Input: part model. Units: mm. Frame: model coordinates. Face numbers are marked on the shaded views. A direction names the side the tool comes from. Give positions to 0.01 mm unless a question says otherwise; leave off trailing zeros. Write each loop counter-clockwise with the first axis right and the second up, starting at its lowest first coordinate (ties: lowest second). Pieces come first, ordered by that corner, then holes.
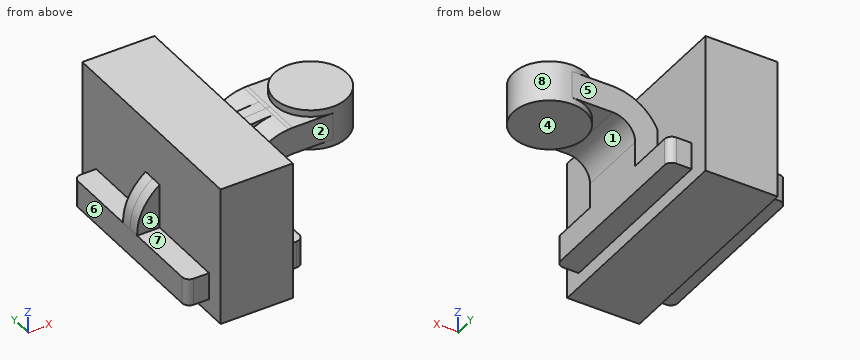
```python
from build123d import *

# Parameters (mm, degrees)
F1_DEPTH = 63.5
F0_W     = 25.4
F0_H     = 19.05
F2_DEPTH = 25.4
F3_DEPTH = 7.9375
F5_R     = 5.08
F6_W     = 155.536965
F6_H     = 98.214656
F7_DEPTH = 25.4


with BuildPart() as f1:
    # F0 (on Front) → F1 (new body, symmetric)
    with BuildSketch(Plane.XZ):
        Polygon((22.225, 9.525), (-41.275, 9.525), (-41.275, -9.525), (41.275, -9.525), (41.275, 9.525), align=None)
    extrude(amount=F1_DEPTH, both=True)

    # F0 (on Front) → F2 (join, symmetric)
    with BuildSketch(Plane.XZ):
        with BuildLine():
            Line((22.225, 27.0002), (22.225, 9.525))
            Line((22.225, 9.525), (41.275, 9.525))
            Line((41.275, 9.525), (41.275, 27.0002))
            ThreePointArc((41.275, 27.0002), (45.92468, 38.22552), (57.15, 42.8752))
            Line((57.15, 42.8752), (60.325, 42.8752))
            Line((60.325, 42.8752), (60.325, 61.9252))
            Line((60.325, 61.9252), (57.15, 61.9252))
            add(Edge.make_bspline(
                [(54.412857, 61.817777), (55.333893, 61.857951), (56.246565, 61.893672), (57.15, 61.9252)],
                knots=[109.005179, 109.005179, 109.005179, 109.005179, 111.504536, 111.504536, 111.504536, 111.504536], degree=3))
            ThreePointArc((54.412857, 61.817777), (31.504822, 50.708436), (22.225, 27.0002))
        make_face()
        with Locations((73.025, 52.4002)):
            Rectangle(F0_W, F0_H)
    extrude(amount=F2_DEPTH, both=True)

    # F0 (on Front) → F3 (join, symmetric)
    with BuildSketch(Plane.XZ):
        with BuildLine():
            add(Edge.make_bspline(
                [(-41.275, 9.525), (-41.833885, 49.842415), (14.243471, 60.065646), (54.412857, 61.817777)],
                knots=[0, 0, 0, 0, 109.005179, 109.005179, 109.005179, 109.005179], degree=3))
            Line((-41.275, 9.525), (22.225, 9.525))
            Line((22.225, 9.525), (22.225, 27.0002))
            ThreePointArc((22.225, 27.0002), (31.504822, 50.708436), (54.412857, 61.817777))
        make_face()
    extrude(amount=F3_DEPTH, both=True)

    # F0 (on Front) → F4 (revolve)
    with BuildSketch(Plane.XZ):
        Polygon((85.725, 66.675), (85.725, 61.9252), (85.725, 42.8752), (85.725, 38.1), (111.125, 38.1), (111.125, 66.675), align=None)
    revolve(axis=Axis((85.725, 0, 52.3875), (0, 0, 1)))

    # F5
    f5_edges = [f1.edges().sort_by_distance(p)[0] for p in [
        (41.275, -63.5, 0),
        (-41.275, -63.5, 0),
        (41.275, 63.5, 0),
        (-41.275, 63.5, 0),
    ]]
    fillet(f5_edges, radius=F5_R)

    # F6 (on Right) → F7 (join, symmetric)
    with BuildSketch(Plane.YZ):
        with Locations((1.350411, 29.165588)):
            Rectangle(F6_W, F6_H)
    extrude(amount=F7_DEPTH, both=True)


solid = f1.part
```
Q1. Access query for the marked faces 1, 2, 3, 4 and 5. Directions: +Z, -Z, +X, -X, +Y, -Y. A direction counts if a zero-diameter tool reaches every point of the face in a straight line with its end or side. Return the directions, or none.
Q2. Mould query, pull axis X, two halves, no side actions, for the marked faces 6, 7 and 8. Classes: +X half, -X half, draft (parallel to the pull), parting line (faces both ways), or undercut.
Q3. Pin query (flat end, axial travel): pin 1 (3 mm diameter, centred on x = -31, z = 2, fed in from +Y); pin 2 (1 mm diameter, centred on y = -41.5, z = 8.5, fed in from -X) (3 decimals); pin 3 (5 mm diameter, centred on x = -31.5, z = 18.5, fed in from -Y). Return the tip coordinate at first contact, or that it passes through.
Q4. Section A-A, the plane y = 56.5. Return the cut outline in (x, z) (3 decimals), then the cut area to 3 significant figures.
Q5. Material intervals for line 1 along Z through (x, y) = (78, 6) (3 decimals); line 2 along X through (y, z) = (39.5, -16); line 3 along X through (y, z) = (-16, 22) (3 decimals), sorted ascending.
Q6. Section B-B, the plane x = 66.5. Return the cut outline in (y, z) (3 decimals), then the cut area to 3 significant figures.
Solutions:
1. face 1: -Z, +Y, -Y
1. face 2: +Z, +X, -Y
1. face 3: +Z, -X, -Y
1. face 4: -Z, +X, +Y, -Y
1. face 5: +Z, +X, +Y
2. face 6: -X half
2. face 7: draft
2. face 8: undercut
3. pin 1: stops at y = 63.5
3. pin 2: stops at x = -41.275
3. pin 3: stops at y = -7.94
4. outline: (-41.275, -9.525) - (-25.4, -9.525) - (-25.4, -19.942) - (25.4, -19.942) - (25.4, -9.525) - (41.275, -9.525) - (41.275, 9.525) - (25.4, 9.525) - (25.4, 78.273) - (-25.4, 78.273) - (-25.4, 9.525) - (-41.275, 9.525) - close
4. area: 5,590 mm2
5. line 1: z = 38.1 to 66.675
5. line 2: x = -25.4 to 25.4
5. line 3: x = -25.4 to 41.275
6. outline: (-25.4, 42.875) - (-16.6, 42.875) - (-16.6, 38.1) - (16.6, 38.1) - (16.6, 42.875) - (25.4, 42.875) - (25.4, 61.925) - (16.6, 61.925) - (16.6, 66.675) - (-16.6, 66.675) - (-16.6, 61.925) - (-25.4, 61.925) - close
6. area: 1,280 mm2
